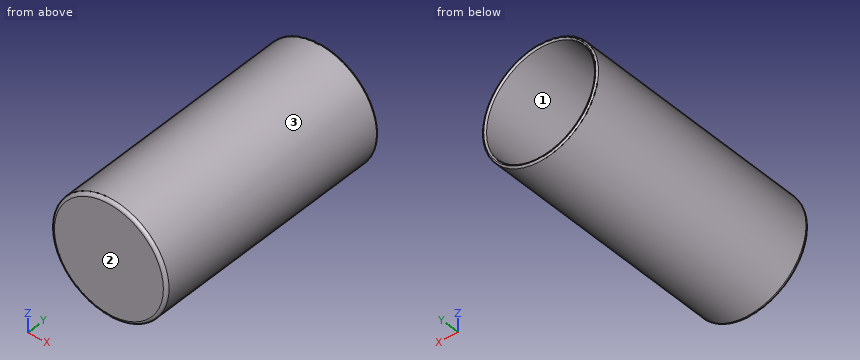
Autodesk Inventor part; units mm, degrees
ref_plane "YZ Plane" through (0, 0, 0) normal (1, 0, 0) x (0, 1, 0)
ref_plane "XZ Plane" through (0, 0, 0) normal (0, 1, 0) x (-1, 0, 0)
ref_plane "XY Plane" through (0, 0, 0) normal (0, 0, 1) x (1, 0, 0)
sketch "Skizze2" plane through (0, 0, 0) normal (0, 1, 0) x (-1, 0, 0)
  circle A0 centre (0, 0) radius 37.5
  dimension "d0" = 75
extrude "Extrusion1" add sketch "Skizze2" along normal blind 160
sketch "Skizze3" plane through (0, 160, 0) normal (0, 1, 0) x (1, 0, 0)
  circle A0 centre (0, 0) radius 35.5
  dimension "d3" = 71
extrude "Extrusion2" cut sketch "Skizze3" against normal blind 150
fillet "Rundung1" radius 1 2 edges at (37.5, 160, 0) (-35.5, 160, 0)
fillet "Rundung2" radius 2 1 edges at (37.5, 0, 0)
fillet "Rundung3" radius 2 1 edges at (-35.5, 10, 0)
properties part number "Glas" material "Glas"
Work out the finished part from the listing and answer in its coordinate system (mm). Face numbers are marked on the shaded views. Coordinates: 2 decimals unless noted, no trailing zeros. Order: outer loops, then holes, each group sorted by start corner. A loop starts at its lowest first (then second) coordinate and runs counter-clockwise, first axis right, second up. Notation, with made-up numbers: (54.5, -9.75) - (60.5, -9.75) arc R24 ccw to (60.5, 18.25) - close; hole circle Ø2 at (56.25, -3). An arc over 180 degrees is marked (long way). Put each result on its own line as item: value. Start each with the question number.
1) Find section B-B (y = 119.5). Give the vertices of the cut face in (x, z).
2) Flat-ended cylindrical pins translate along their axes: pin 1 (4 mm diameter, centred on x = -6.5, z = 11, fed in from -Y); pin 2 (10 mm diameter, centred on x = 14, z = -14.5, fed in from +Y); pin 3 (6 mm diameter, centred on y = 66, z = 19, fed in from +X); pin 4 (1.5 mm diameter, centred on x = 4, y = 45.5, fed in from -Z). Find the tip coordinate at first contact, or state that the pin passes through.
3) Find the intervals of material crossed by line 1 (X direction, y = 50.5, z = -1); line 2 (Z direction, x = 0, y = 84.5); line 3 (Y direction, x = -16, z = 24), in increasing order. Write a range as from..to.
4) For a pull along Z with two mould halves and no side action, classify the marked faces 1, 2 and 3 as released by +Z, released by -Z, zero draft, split by the parting line, or undercut.
Results list:
1. outline: circle Ø75 at (0, 0); hole circle Ø71 at (0, 0)
2. pin 1: stops at y = 0
2. pin 2: stops at y = 10
2. pin 3: stops at x = 33.92
2. pin 4: stops at z = -37.36
3. line 1: x = -37.49..-35.49, 35.49..37.49
3. line 2: z = -37.5..-35.5, 35.5..37.5
3. line 3: y = 0..10
4. face 1: undercut
4. face 2: zero draft
4. face 3: split by the parting line
